Autodesk Inventor part; units mm, degrees
ref_plane "YZ Plane" through (0, 0, 0) normal (1, 0, 0) x (0, 1, 0)
ref_plane "XZ Plane" through (0, 0, 0) normal (0, 1, 0) x (-1, 0, 0)
ref_plane "XY Plane" through (0, 0, 0) normal (0, 0, 1) x (1, 0, 0)
sketch "Эскиз1" plane through (0, 0, 0) normal (0, 0, 1) x (1, 0, 0)
  circle A0 centre (0, 0) radius 30
  circle A1 centre (0, 0) radius 45
  dimension "d0" = 60
  dimension "d1" = 90
extrude "Выдавливание1" add sketch "Эскиз1" along normal blind 5
sketch "Эскиз2" plane through (0, 0, 0) normal (1, 0, 0) x (0, 1, 0)
  line L0 (-45, 0) -> (-45, 5)
  line L1 (0, -0.8) -> (0, 4.8)
  line L2 (-45, 0) -> (-45, 5)
  line L3 (-45, 2.5) -> (-44, 2.5)
  circle A0 centre (-44, 2.5) radius 1
  line L4 (-44, 3.5) -> (-45, 3.5)
  line L5 (-44, 1.5) -> (-45, 1.5)
  line L6 (-45, 0) -> (-45, 5)
  point P0 (0, 0)
  dimension "d6" = 1
  dimension "d7" = 2
revolve "Вращение1" cut sketch "Эскиз2" angle 360 about axis through (0, 0, -10) along (0, 0, 1)
sketch "Эскиз3" plane through (0, 0, 0) normal (1, 0, 0) x (0, 1, 0)
  line L0 (45, 0) -> (-45, 0)
  line L1 (30, 0) -> (30, -2.5)
  line L2 (30, -2.5) -> (34, -2.5)
  line L3 (34, -2.5) -> (36.5, 0)
  line L4 (0, -4) -> (0, 6.5)
  point P0 (0, 0)
  dimension "d9" = 2.5
  dimension "d10" = 4
  dimension "d11" = 135
revolve "Вращение2" add sketch "Эскиз3" angle 360 about axis through (0, 0, -10) along (0, 0, 1)
properties part number "Кольцо сальника 1" material "Сталь, легированная"
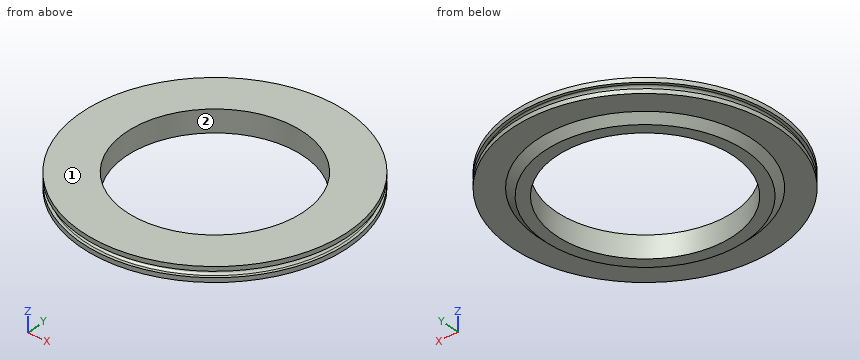
CAD build for the part. Positions are in the model's coordinates, mm. Face numbers are marked on the shaded views. Round coordinates to 2 decimals unless told otherwise and drop trailing zeros. Loops run counter-clockwise (first coordinate to the right, second up) from the corner with the lowest first, then second, coordinate; pieces in that order, holes last. Notation, with made-up numbers: M 4,-33 L 53,-33 A15 cw 53,-12 Z; hole C 42.5,66 d8. An arc over 180 degrees is marked long. Return JSON: item names as keys, results as strings. Group by question number.
(1) Mould opens along X. For the marked faces 1 and 2 say: +X half, -X half, draft (parallel to the pull), parting line (faces both ways), or undercut.
(2) Drop flat-ended pins along their axis: P1, Ø4, axis at x = 18, z = -1.5, coming from the -Y side; P2, Ø2, axis at x = -7.5, z = 4, coming from the +Y side; P3, Ø1.5, axis at y = 14.5, z = 3, coming from the -X side. Give the stop position or say it passes through.
(3) Wall check: probe 1 along Y at (x, z) = (0, 1); probe 2 along Y at (x, z) = (-26.5, -1). Give the ranges that are in metal, low to high. Write a range as [from, to].
(4) Saw through at A-A, the plane x = 0. List the corners of the cut face in (y, z), and give its area (3 significant figures).
Answer list:
{
 "1": {"face 1": "draft", "face 2": "undercut"},
 "2": {"P1": "y = -41.8", "P2": "y = 44.53", "P3": "x = -42.79"},
 "3": {"probe 1": "[-45, -30], [30, 45]", "probe 2": "[-23.62, -14.06], [14.06, 23.62]"},
 "4": {"outline": "M -45,0 L -36.5,0 L -34,-2.5 L -30,-2.5 L -30,5 L -45,5 L -45,3.5 L -44,3.5 A1 cw -44,1.5 L -45,1.5 Z; M 30,-2.5 L 34,-2.5 L 36.5,0 L 45,0 L 45,1.5 L 44,1.5 A1 cw 44,3.5 L 45,3.5 L 45,5 L 30,5 Z", "area": "169 mm2"}
}
